Geometry: final body of the model. Coordinates: model frame, mm. Coordinates: 2 decimals unless noted, no trailing zeros. Order: outer loops, then holes, each group sorted by start corner. A loop starts at its lowest first (then second) coordinate and runs counter-clockwise, first axis right, second up. Notation, with made-up numbers: (4, 20.25) -> (60, 20.25) arc R9 cw to (60, 28.25) -> close; hole circle Ø3 at (33, 75). An arc over 180 degrees is marked (long way). Answer in a Markdown table with one row per item. Add a question column.
1) Section query C-C on x = 5.75. Return the cut outline in (y, z), then the cut area to 3 significant figures.
2) Section query A-A on z = 80. Return the cut outline in (x, y), then the cut area to 3 significant figures.
3) Ray query, line 1 (Z direction, x = 6, y = 25); line 2 (Y direction, x = 5.25, z = 20); line 3 (Y direction, x = 6.25, z = 18). Return the intervals inside material, ascending. Write a range as from..to.
4) Pull-direction query (Y, two-part tool) for faces 1 (the face through (5, 50, 49)), 2 (the face through (5, 0, 51)), 3 (the face through (4.93, 23.92, 84.88)); classes: +Y half, -Y half, draft (parallel to the pull), parting line (faces both ways), or undercut.
5) Section query B-B on y = 25. Return the cut outline in (x, z), then the cut area to 3 significant figures.
Autodesk Inventor part; units mm, degrees
ref_plane "YZ Plane" through (0, 0, 0) normal (1, 0, 0) x (0, 1, 0)
ref_plane "XZ Plane" through (0, 0, 0) normal (0, 1, 0) x (-1, 0, 0)
ref_plane "XY Plane" through (0, 0, 0) normal (0, 0, 1) x (1, 0, 0)
sketch "Sketch1" plane through (0, 0, 0) normal (1, 0, 0) x (0, 1, 0)
  line L0 (0, 0) -> (50, 0)
  line L1 (50, 0) -> (50, 100)
  line L2 (50, 100) -> (0, 100)
  line L3 (0, 100) -> (0, 0)
  line L4 (25, 108.4087) -> (25, -21.5037)
  circle A0 centre (25, 80) radius 5
  line L5 (63.0593, 50) -> (-7.0373, 50)
  circle A1 centre (25, 20) radius 5
  dimension "d0" = 100
  dimension "d1" = 50
  dimension "d4" = 25
  dimension "d5" = 20
  dimension "d6" = 50
  dimension "d9" = 10
extrude "Extrusion2" add sketch "Sketch1" along normal blind 10 contours L3 L5 L4 A1 L0 | L4 A1 L5 L1 L0 | L3 L2 L4 A0 L5 | L4 A0 L2 L1 L5
equation "\"d4\" = 0.5 * d1"
equation "\"d5\" = 0.2 * d0"
equation "\"d6\" = 0.5 * d0"
properties part number "block"
Result:
| question | item | result |
|---|---|---|
| 1 | outline | (0, 0) -> (50, 0) -> (50, 100) -> (0, 100) -> close; hole circle Ø10 at (25, 20); hole circle Ø10 at (25, 80) |
| 1 | area | 4,840 mm2 |
| 2 | outline | (0, 0) -> (10, 0) -> (10, 20) -> (0, 20) -> close; (0, 30) -> (10, 30) -> (10, 50) -> (0, 50) -> close |
| 2 | area | 400 mm2 |
| 3 | line 1 | 0..15, 25..75, 85..100 |
| 3 | line 2 | 0..20, 30..50 |
| 3 | line 3 | 0..20.42, 29.58..50 |
| 4 | face 1 | +Y half |
| 4 | face 2 | -Y half |
| 4 | face 3 | undercut |
| 5 | outline | (0, 0) -> (10, 0) -> (10, 15) -> (0, 15) -> close; (0, 25) -> (10, 25) -> (10, 75) -> (0, 75) -> close; (0, 85) -> (10, 85) -> (10, 100) -> (0, 100) -> close |
| 5 | area | 800 mm2 |
